from build123d import *

# Parameters (mm, degrees)
SKETCH1_R               = 46.5
BOSS_EXTRUDE1_DEPTH     = 30
SKETCH1_3_R             = 55
SKETCH1_3_R_2           = 46.5
BOSS_EXTRUDE2_DEPTH     = 8
CUT_EXTRUDE1_DEPTH      = 81.833161512
CUT_EXTRUDE1_DEPTH_BACK = 81.833161512
SKETCH2_R               = 2.5
SKETCH3_R               = 44.5
CUT_EXTRUDE2_DEPTH      = 22


with BuildPart() as part:
    # Sketch1 → Boss-Extrude1 (new body)
    with BuildSketch(Plane.XY):
        Circle(SKETCH1_R)
    extrude(amount=BOSS_EXTRUDE1_DEPTH)

    # Sketch1<3> → Boss-Extrude2 (add)
    with BuildSketch(Plane.XY):
        Circle(SKETCH1_3_R)
        Circle(SKETCH1_3_R_2, mode=Mode.SUBTRACT)
    extrude(amount=BOSS_EXTRUDE2_DEPTH)

    # Sketch2 → Cut-Extrude1 (cut, two sides: drawn at the far end of the back side and taken through both)
    with BuildSketch(Plane.XY.offset(8).offset(-CUT_EXTRUDE1_DEPTH_BACK)):
        with Locations((0, 51)):
            Circle(SKETCH2_R)
        with Locations((0, -51)):
            Circle(SKETCH2_R)
    extrude(amount=CUT_EXTRUDE1_DEPTH + CUT_EXTRUDE1_DEPTH_BACK, mode=Mode.SUBTRACT)

    # Sketch3 → Cut-Extrude2 (cut)
    with BuildSketch(Plane.XY.offset(30)):
        Circle(SKETCH3_R)
    extrude(amount=-CUT_EXTRUDE2_DEPTH, mode=Mode.SUBTRACT)


solid = part.part
For this review, take the finished solid that the model builds, in its own axes (mm). A direction names the side the tool comes from. Round coordinates to 2 decimals unless told otherwise and drop trailing zeros. Write each loop counter-clockwise with the first axis right and the second up, starting at its lowest first coordinate (ties: lowest second). Pieces come first, ordered by that corner, then holes. Notation, with made-up numbers: (33.25, 46.25) -> (88.25, 46.25) arc R17 ccw to (88.25, 60.25) -> close; hole circle Ø9 at (-38, -15.75). An arc over 180 degrees is marked (long way). Use CSV: the item, a comma, the result in double quotes.
(1) Draft analysis for pull direction Y (two halves, no side actions). For faces 1 (the face through (-1, 1, 8)), 2 (the face through (44.35, 13.97, 18.85)), 3 (the face through (12, 45.1, 8)), state which applies: +Y half, -Y half, draft (parallel to the pull), parting line (faces both ways), or undercut.
Computed values:
face 1,"undercut"
face 2,"parting line"
face 3,"draft"
(2) Clearance check with flat-ended pins moving along their axes: P1, Ø6.5, axis at x = 0, y = -51, coming from the +Z side; P2, Ø4, axis at x = 26, z = 20.5, coming from the -Y side; P3, Ø12, axis at y = -36.5, z = 18, coming from the -X side. State where each tip first meets the part, or that it passes through.
Computed values:
P1,"z = 8"
P2,"y = -39.83"
P3,"x = -35.1"
(3) For faces 4 (the face through (-0.54, 48.56, 3.94)), 5 (the face through (-32.798, 30.075, 19.154)), list the 3-axis set-ups (+Z, -Z, +X, -X, +Y, -Y) from which the entire face can be reached by the end or side of a thin tool; tool diameter is ignored.
Computed values:
face 4,"+Z, -Z"
face 5,"+Z"
(4) To check wall thickness, follow L1, parallel to Y at x = 0, z = 5.25; L2, parallel to Y at x = 0, z = 23.25; L3, parallel to Z at x = -40.5, y = 3.5. State the ranges of each line that lie inside material, in increasing order. Write a range as [from, to].
Computed values:
L1,"[-55, -53.5], [-48.5, 48.5], [53.5, 55]"
L2,"[-46.5, -44.5], [44.5, 46.5]"
L3,"[0, 8]"
(5) Consider section A-A, the plane x = 0. Give the boundary of the cut face in (y, z).
Computed values:
outline,"(-55, 0) -> (-53.5, 0) -> (-53.5, 8) -> (-55, 8) -> close; (-48.5, 0) -> (48.5, 0) -> (48.5, 8) -> (46.5, 8) -> (46.5, 30) -> (44.5, 30) -> (44.5, 8) -> (-44.5, 8) -> (-44.5, 30) -> (-46.5, 30) -> (-46.5, 8) -> (-48.5, 8) -> close; (53.5, 0) -> (55, 0) -> (55, 8) -> (53.5, 8) -> close"
(6) Consider section B-B, the plane y = -51. Give the boundary of the cut face in (x, z).
Computed values:
outline,"(-20.59, 0) -> (-2.5, 0) -> (-2.5, 8) -> (-20.59, 8) -> close; (2.5, 0) -> (20.59, 0) -> (20.59, 8) -> (2.5, 8) -> close"
(7) Consider section C-C, the plane y = 0. Give the boundary of the cut face in (x, z), plus the area to 3 significant figures.
Computed values:
outline,"(-55, 0) -> (55, 0) -> (55, 8) -> (46.5, 8) -> (46.5, 30) -> (44.5, 30) -> (44.5, 8) -> (-44.5, 8) -> (-44.5, 30) -> (-46.5, 30) -> (-46.5, 8) -> (-55, 8) -> close"
area,"968 mm²"
(8) Consider section D-D, the plane z = 4. Give the boundary of the cut face in (x, y).
Computed values:
outline,"circle Ø110 at (0, 0); hole circle Ø5 at (0, -51); hole circle Ø5 at (0, 51)"
